Geometry check sheet. Reference: the model listing, model coordinates, mm. Round coordinates to 2 decimals unless told otherwise and drop trailing zeros.
```python
from build123d import *

# Parameters (mm, degrees)
F0_W     = 63
F0_H     = 75
F1_DEPTH = 500
F2_SIZE  = 5
F3_R     = 4
F4_DEPTH = 63.001


with BuildPart() as f1:
    # F0 (on Front) → F1 (new body)
    with BuildSketch(Plane.XZ):
        Rectangle(F0_W, F0_H)
    extrude(amount=F1_DEPTH)

    # F2
    f2_edges = [f1.edges().sort_by_distance(p)[0] for p in [
        (31.5, -250, -37.5),
        (-31.5, -250, -37.5),
    ]]
    chamfer(f2_edges, length=F2_SIZE)

    # F3 (on face) → F4 (cut, through all)
    with BuildSketch(Plane.YZ.offset(31.5)):
        with Locations((-470, -17.5)):
            Circle(F3_R)
    extrude(amount=-F4_DEPTH, mode=Mode.SUBTRACT)


solid = f1.part
```
1) Gauge pin test, flat end, axial feed: pin 1 (6 mm diameter, centred on x = -22.5, z = 7.5, fed in from +Y). Record the tip position at first contact, or that the pin passes through.
Report:
pin 1: stops at y = 0
2) Scan lines: line 1 along Z through (x, y) = (-12, -470); line 2 along Y through (x, z) = (1, -17); line 3 along Z through (x, y) = (27, -254). Record each from-to range of solid material in increasing order.
Report:
line 1: z = -37.5 to -21.5, -13.5 to 37.5
line 2: y = -500 to -473.97, -466.03 to 0
line 3: z = -37 to 37.5
3) Mould release check, pull along Z, two halves, no side actions. Record for faces 1 (the face through (0, -500, 1)), 2 (the face through (0.441, -473.996, -17.324)), 3 (the face through (0, -246, 37.5)): +Z half, -Z half, draft (parallel to the pull), parting line (faces both ways), or undercut.
Report:
face 1: draft
face 2: undercut
face 3: +Z half
